CAD build for the part. Positions are in the model's coordinates, mm. Face numbers are marked on the shaded views. A direction names the side the tool comes from. Give positions to 0.01 mm unless a question says otherwise; leave off trailing zeros. Write each loop counter-clockwise with the first axis right and the second up, starting at its lowest first coordinate (ties: lowest second). Pieces come first, ordered by that corner, then holes. Notation, with made-up numbers: (23.25, 86.5) -> (70.25, 86.5) arc R38 ccw to (70.25, 124.5) -> close; hole circle Ø10 at (2.25, -5.75). An arc over 180 degrees is marked (long way). Answer in a Markdown table with one row per item. Add a question column.
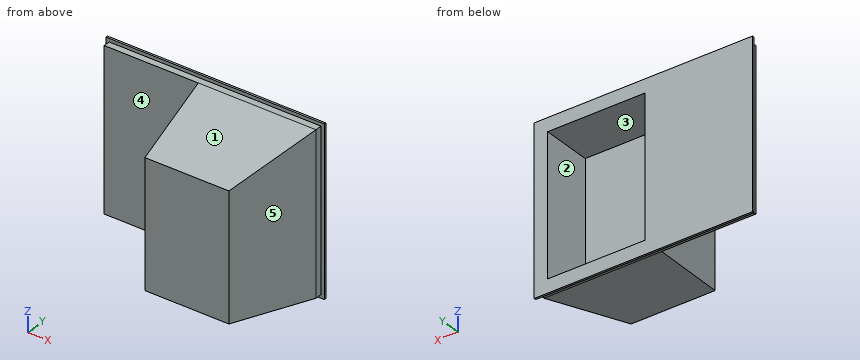
```python
from build123d import *

# Parameters (mm, degrees)
SKETCH_1_W               = 630
SKETCH_1_H               = 475
EXTRUDE_1_DEPTH          = 300
CUT_EXTRUDE_1_DEPTH      = 1
CUT_EXTRUDE_1_DEPTH_BACK = 476
SKETCH_3_W               = 650
SKETCH_3_H               = 495
EXTRUDE_2_DEPTH          = 6
CUT_EXTRUDE_2_DEPTH      = 11
CUT_EXTRUDE_2_DEPTH_BACK = 641
SKETCH_5_W               = 290
SKETCH_5_H               = 415
CUT_EXTRUDE_4_DEPTH      = 150


with BuildPart() as part:
    # Эскиз1 → Бобышка-Вытянуть1 (new body)
    with BuildSketch(Plane(origin=(0, 0, 0), x_dir=(1, 0, 0), z_dir=(0, 1, 0))):
        Rectangle(SKETCH_1_W, SKETCH_1_H)
    extrude(amount=EXTRUDE_1_DEPTH)

    # Эскиз2 → Вырез-Вытянуть1 (cut, two sides)
    with BuildSketch(Plane.XY.offset(237.5)) as cut_extrude_1_sk:
        Polygon((-315, 0), (15, 0), (-35, 280), (-315, 280), align=None)
        Polygon((315, 280), (265, 0), (315, 0), align=None)
    extrude(amount=CUT_EXTRUDE_1_DEPTH, mode=Mode.SUBTRACT)
    extrude(cut_extrude_1_sk.sketch, amount=-CUT_EXTRUDE_1_DEPTH_BACK, mode=Mode.SUBTRACT)

    # Эскиз3 → Бобышка-Вытянуть2 (add)
    with BuildSketch(Plane(origin=(0, 300, 0), x_dir=(1, 0, 0), z_dir=(0, 1, 0))):
        Rectangle(SKETCH_3_W, SKETCH_3_H)
    extrude(amount=EXTRUDE_2_DEPTH)

    # Эскиз4 → Вырез-Вытянуть2 (cut, two sides)
    with BuildSketch(Plane(origin=(315, 0, 0), x_dir=(0, 0, -1), z_dir=(1, 0, 0))) as cut_extrude_2_sk:
        Polygon((-237.5, 280), (-187.5, 0), (-237.5, 0), align=None)
        Polygon((237.5, 280), (237.5, 0), (187.5, 0), align=None)
    extrude(amount=CUT_EXTRUDE_2_DEPTH, mode=Mode.SUBTRACT)
    extrude(cut_extrude_2_sk.sketch, amount=-CUT_EXTRUDE_2_DEPTH_BACK, mode=Mode.SUBTRACT)

    # Эскиз5 → Вырез-Вытянуть4 (cut)
    with BuildSketch(Plane(origin=(0, 306, 0), x_dir=(1, 0, 0), z_dir=(0, 1, 0))):
        with Locations((140, 0)):
            Rectangle(SKETCH_5_W, SKETCH_5_H)
    extrude(amount=-CUT_EXTRUDE_4_DEPTH, mode=Mode.SUBTRACT)


solid = part.part
```
Item 1: Slice it at D-D, the plane z = -180. List the corners of the cut face in (x, y).
Item 2: Slice it at B-B, the plane x = -275. List the corners of the cut face in (y, z), then the cut area to 3 significant figures.
Item 3: Probe L1, parallel to Y at x = -157, z = 95; L2, parallel to X at y = 167, z = 177; L3, parallel to Z at x = 60, y = 240. List the from-to ranges inside material, lowest first. Write a range as from..to.
Item 4: Slice it at A-A, the plane z = 216. List the corners of the cut face in (x, y), then the cut area to 3 significant figures.
Item 5: Which spindle directions (+Z, -Z, +X, -X, +Y, -Y) get a long thin tool onto all of the face, cutting with end or side? Do the marked faces 1 and 2. Say none if no direction does.
Item 6: Drop flat-ended pins along their axis: pin 1 Ø10 at (x, z) = (-110.5, -33) entering from -Y; pin 2 Ø5 at (x, z) = (234.5, 36) entering from -Y; pin 3 Ø10 at (x, y) = (-15, 289) entering from +Z; pin 4 Ø10 at (x, y) = (-96, 288.5) entering from -Z. Give the stop position or say it passes through.
Item 7: Mould opens along X. For the marked faces 3, 4 and 5 say: released by +X, released by -X, zero draft, split by the parting line, or undercut.
Item 8: Slice it at C-C, the plane y = 186.5. List the corners of the cut face in (x, z).
Answer key:
| question | item | result |
|---|---|---|
| 1 | outline | (-325, 300) -> (-315, 300) -> (-315, 280) -> (-35, 280) -> (15, 0) -> (265, 0) -> (315, 280) -> (315, 300) -> (325, 300) -> (325, 306) -> (285, 306) -> (285, 156) -> (-5, 156) -> (-5, 306) -> (-325, 306) -> close |
| 2 | outline | (280, -237.5) -> (300, -237.5) -> (300, -247.5) -> (306, -247.5) -> (306, 247.5) -> (300, 247.5) -> (300, 237.5) -> (280, 237.5) -> close |
| 2 | area | 12,500 mm² |
| 3 | L1 | y = 280..306 |
| 3 | L2 | x = -14.82..-5, 285..294.82 |
| 3 | L3 | z = -230.36..-207.5, 207.5..230.36 |
| 4 | outline | (-325, 300) -> (-315, 300) -> (-315, 280) -> (-35, 280) -> (-13.5, 159.6) -> (293.5, 159.6) -> (315, 280) -> (315, 300) -> (325, 300) -> (325, 306) -> (-325, 306) -> close |
| 4 | area | 56,100 mm² |
| 5 | face 1 | +Z, +X, -X, -Y |
| 5 | face 2 | +Y |
| 6 | pin 1 | stops at y = 280 |
| 6 | pin 2 | stops at y = 0 |
| 6 | pin 3 | stops at z = 237.5 |
| 6 | pin 4 | stops at z = -237.5 |
| 7 | face 3 | undercut |
| 7 | face 4 | zero draft |
| 7 | face 5 | released by +X |
| 8 | outline | (-18.3, -220.8) -> (298.3, -220.8) -> (298.3, 220.8) -> (-18.3, 220.8) -> close; hole (-5, -207.5) -> (285, -207.5) -> (285, 207.5) -> (-5, 207.5) -> close |
